```python
from build123d import *

# Parameters (mm, degrees)
EXTRUDE_1_DEPTH     = 5
CUT_EXTRUDE_1_REACH = 7
SKETCH_2_W          = 19.790240303
SKETCH_2_H          = 15
SKETCH_2_W_2        = 23.6545041
CUT_EXTRUDE_2_REACH = 7
SKETCH_3_W          = 5
SKETCH_3_H          = 5


with BuildPart() as part:
    # 草图1 → 凸台-拉伸1 (new body)
    with BuildSketch(Plane.XY):
        Polygon((0, 0), (-98.660254038, 0), (-90, 15), (-30, 15), (-30, 20), (-60, 20), (58.356805184, 225), (104.919223085, 225), align=None)
    extrude(amount=EXTRUDE_1_DEPTH)

    # 草图2 → 切除-拉伸1 (cut, up to next)
    with BuildSketch(Plane.XY.offset(5), mode=Mode.PRIVATE) as cut_extrude_1_sk1:
        with Locations((104.814343237, 217.5)):
            Rectangle(SKETCH_2_W, SKETCH_2_H)
    cut_extrude_1_tool1 = extrude(cut_extrude_1_sk1.sketch, amount=-CUT_EXTRUDE_1_REACH, mode=Mode.PRIVATE) & part.part
    add(cut_extrude_1_tool1.solids().sort_by_distance((104.814343, 217.5, 5))[0], mode=Mode.SUBTRACT)
    # 草图2 → 切除-拉伸1 (cut, up to next)
    with BuildSketch(Plane.XY.offset(5), mode=Mode.PRIVATE) as cut_extrude_1_sk2:
        with Locations((58.091971035, 217.5)):
            Rectangle(SKETCH_2_W_2, SKETCH_2_H)
    cut_extrude_1_tool2 = extrude(cut_extrude_1_sk2.sketch, amount=-CUT_EXTRUDE_1_REACH, mode=Mode.PRIVATE) & part.part
    add(cut_extrude_1_tool2.solids().sort_by_distance((58.091971, 217.5, 5))[0], mode=Mode.SUBTRACT)

    # 草图3 → 切除-拉伸2 (cut, up to next)
    with BuildSketch(Plane.XY.offset(5), mode=Mode.PRIVATE) as cut_extrude_2_sk1:
        with Locations((72.419223085, 217.5)):
            Rectangle(SKETCH_3_W, SKETCH_3_H)
    cut_extrude_2_tool1 = extrude(cut_extrude_2_sk1.sketch, amount=-CUT_EXTRUDE_2_REACH, mode=Mode.PRIVATE) & part.part
    add(cut_extrude_2_tool1.solids().sort_by_distance((72.419223, 217.5, 5))[0], mode=Mode.SUBTRACT)
    # 草图3 → 切除-拉伸2 (cut, up to next)
    with BuildSketch(Plane.XY.offset(5), mode=Mode.PRIVATE) as cut_extrude_2_sk2:
        with Locations((92.419223085, 217.5)):
            Rectangle(SKETCH_3_W, SKETCH_3_H)
    cut_extrude_2_tool2 = extrude(cut_extrude_2_sk2.sketch, amount=-CUT_EXTRUDE_2_REACH, mode=Mode.PRIVATE) & part.part
    add(cut_extrude_2_tool2.solids().sort_by_distance((92.419223, 217.5, 5))[0], mode=Mode.SUBTRACT)


solid = part.part
```
Check sheet for the modelled part. Datum: model origin and axes. Units: mm. A direction names the side the tool comes from. Round coordinates to 2 decimals unless told otherwise and drop trailing zeros. Order: outer loops, then holes, each group sorted by start corner. A loop starts at its lowest first (then second) coordinate and runs counter-clockwise, first axis right, second up. Notation, with made-up numbers: (-4.75, 32) -> (33.25, 32) arc R26 cw to (33.25, 66) -> close; hole circle Ø5 at (37, -39.75). An arc over 180 degrees is marked (long way). One line per item, written item: value. Start each with the question number.
Q1. Cross-section at A-A (x = -56.5). Record the boundary of the cut face in (y, z), and give its area (3 significant figures).
Q2. Cross-section at B-B (z = 4.1). Record the boundary of the cut face in (x, y).
Q3. Thickness scan on line 1 (Y direction, x = -81.5, z = 0.4); line 2 (Y direction, x = -48.5, z = 4.05); line 3 (X direction, y = 195.5, z = 4.05). Record the ranges inside material, lowest first.
Q4. Mould release check, pull along Y, two halves, no side actions. Record for faces 1 (the face through (92, 220, 3)), 2 (the face through (69.919, 212, 3)), 3 (the face through (-60, 15, 2)), 4 (the face through (82, 225, 2)): pulls with the +Y half, pulls with the -Y half, needs draft (parallel to the pull), parting line crosses it, or undercut.
Q5. Cross-section at C-C (x = -76.5). Record the boundary of the cut face in (y, z), and give its area (3 significant figures).
Q6. Cross-section at D-D (y = 188). Record the boundary of the cut face in (x, z), and give its area (3 significant figures).
Q7. Set-up check for faces 5 (the face through (89.919, 217, 3)), 6 (the face through (94.919, 212, 3)), 7 (the face through (74.919, 217, 3)), 8 (the face through (69.919, 222, 3)): record each of +Z, -Z, +X, -X, +Y, -Y from which the full face is reachable in a straight line by a thin tool's end or side.
Q8. Gauge pin test, flat ends, axial feed: pin 1 Ø2.5 at (x, z) = (93.5, 2) entering from -Y; pin 2 Ø1.5 at (y, z) = (216.5, 3.5) entering from +X; pin 3 Ø2.5 at (x, z) = (71, 2.5) entering from -Y. Record the tip position at first contact, or that the pin passes through.
Completed:
1. outline: (0, 0) -> (15, 0) -> (15, 5) -> (0, 5) -> close; (20, 0) -> (26.06, 0) -> (26.06, 5) -> (20, 5) -> close
1. area: 105 mm²
2. outline: (-98.66, 0) -> (0, 0) -> (97.92, 210) -> (94.92, 210) -> (94.92, 215) -> (89.92, 215) -> (89.92, 220) -> (94.92, 220) -> (94.92, 225) -> (69.92, 225) -> (69.92, 220) -> (74.92, 220) -> (74.92, 215) -> (69.92, 215) -> (69.92, 210) -> (49.7, 210) -> (-60, 20) -> (-30, 20) -> (-30, 15) -> (-90, 15) -> close
3. line 1: y = 0 to 15
3. line 2: y = 0 to 15, 20 to 39.92
3. line 3: x = 41.32 to 91.16
4. face 1: undercut
4. face 2: needs draft
4. face 3: undercut
4. face 4: pulls with the +Y half
5. outline: (0, 0) -> (15, 0) -> (15, 5) -> (0, 5) -> close
5. area: 75.0 mm²
6. outline: (36.99, 0) -> (87.67, 0) -> (87.67, 5) -> (36.99, 5) -> close
6. area: 253 mm²
7. face 5: +Z, -Z, +X
7. face 6: +Z, -Z, +X, +Y
7. face 7: +Z, -Z, -X
7. face 8: +Z, -Z, -X, +Y
8. pin 1: stops at y = 197.83
8. pin 2: stops at x = 89.92
8. pin 3: stops at y = 149.58
